For this review, take the finished solid that the model builds, in its own axes (mm). Round coordinates to 2 decimals unless told otherwise and drop trailing zeros. Order: outer loops, then holes, each group sorted by start corner. A loop starts at its lowest first (then second) coordinate and runs counter-clockwise, first axis right, second up. Notation, with made-up numbers: M 78,-15.5 L 95,-15.5 A22 ccw 95,-7.5 Z; hole C 68.5,28.5 d8. An arc over 180 degrees is marked long. Use a Markdown table: item, result.
from build123d import *

# Parameters (mm, degrees)
BOSS_EXTRUDE1_DEPTH = 0.375


with BuildPart() as part:
    # Sketch1 → Revolve1 (revolve)
    with BuildSketch(Plane.XY):
        with BuildLine():
            Line((0.25, 0.226271737), (0.25, 46))
            Line((0.25, 46), (0, 46))
            Line((0, 46), (0, -0.337192673))
            ThreePointArc((0, -0.337192673), (0.308217513, -0.136751101), (0.25, 0.226271737))
        make_face()
    revolve(axis=Axis((0, 46, 0), (0, -1, 0)))

    # Sketch3 → Boss-Extrude1 (add, symmetric)
    with BuildSketch(Plane(origin=(0, 0, 0), x_dir=(0, 0, -1), z_dir=(1, 0, 0))):
        with BuildLine():
            Line((1.25, 44.5), (1.25, 45.25))
            ThreePointArc((1.25, 45.25), (1.030330086, 45.780330086), (0.5, 46))
            Line((0.5, 46), (-0.5, 46))
            ThreePointArc((-0.5, 46), (-1.030330086, 45.780330086), (-1.25, 45.25))
            Line((-1.25, 45.25), (-1.25, 44.5))
            ThreePointArc((-1.25, 44.5), (-0.95772294, 41.553326298), (-0.092281879, 38.721485279))
            ThreePointArc((-0.092281879, 38.721485279), (0, 38.660008711), (0.092281879, 38.721485279))
            ThreePointArc((0.092281879, 38.721485279), (0.95772294, 41.553326298), (1.25, 44.5))
        make_face()
    extrude(amount=BOSS_EXTRUDE1_DEPTH, both=True)


solid = part.part
Q1. Wall thickness on line 1 along Z through (x, y) = (0, 44); line 2 along Z through (x, y) = (-0.1, 12): over which ranges is each line inside the solid? List them lowest first. Write a range as [from, to].
Determined:
| item | result |
|---|---|
| line 1 | z = [-1.24, 1.24] |
| line 2 | z = [-0.23, 0.23] |
Q2. Add section B-B (y = 27). Write out the cut boundary in (x, z).
Determined:
| item | result |
|---|---|
| outline | C 0,0 d0.5 |
Q3. Add section A-A (x = 0). Write out the cut boundary in (y, z), then the cut area to 3 significant figures.
Determined:
| item | result |
|---|---|
| outline | M 0.23,-0.25 L 39.11,-0.25 A15 ccw 44.5,-1.25 L 45.25,-1.25 A0.75 ccw 46,-0.5 L 46,0.5 A0.75 ccw 45.25,1.25 L 44.5,1.25 A15 ccw 39.11,0.25 L 0.23,0.25 A0.34 ccw long Z |
| area | 33.2 mm^2 |
Q4. Add section C-C (y = 41). Write out the cut boundary in (x, z) (3 decimals), then the cut area to 3 significant figures.
Determined:
| item | result |
|---|---|
| outline | M -0.375,-0.836 L 0.375,-0.836 L 0.375,0.836 L -0.375,0.836 Z |
| area | 1.25 mm^2 |
